```python
from build123d import *

# Parameters (mm, degrees)
Y_KSEKLIK_EKSTR_ZYON1_DEPTH = 500
RADYUS1_R                   = 2
IZIM2_R                     = 4.25
KES_EKSTR_ZYON1_DEPTH       = 10


with BuildPart() as part:
    # Çizim1 → Yükseklik-Ekstrüzyon1 (new body)
    with BuildSketch(Plane.XY):
        Polygon((0, 0), (65, 0), (65, 4), (60, 4), (60, 8), (55, 8), (55, 4), (10, 4), (10, 8), (5, 8), (5, 4), (0, 4), align=None)
    extrude(amount=-Y_KSEKLIK_EKSTR_ZYON1_DEPTH)

    # Radyus1
    radyus1_edges = [part.edges().sort_by_distance(p)[0] for p in [
        (5, 8, -250),
        (10, 8, -250),
        (55, 8, -250),
        (60, 8, -250),
    ]]
    fillet(radyus1_edges, radius=RADYUS1_R)

    # Çizim2 → Kes-Ekstrüzyon1 (cut)
    with BuildSketch(Plane.XZ):
        with Locations(Location((30, -40, 0), (0, 0, 270))):
            Circle(IZIM2_R)
        with Locations(Location((30, -180, 0), (0, 0, 270))):
            Circle(IZIM2_R)
        with Locations(Location((30, -320, 0), (0, 0, 270))):
            Circle(IZIM2_R)
        with Locations(Location((30, -460, 0), (0, 0, 270))):
            Circle(IZIM2_R)
    extrude(amount=-KES_EKSTR_ZYON1_DEPTH, mode=Mode.SUBTRACT)


solid = part.part
```
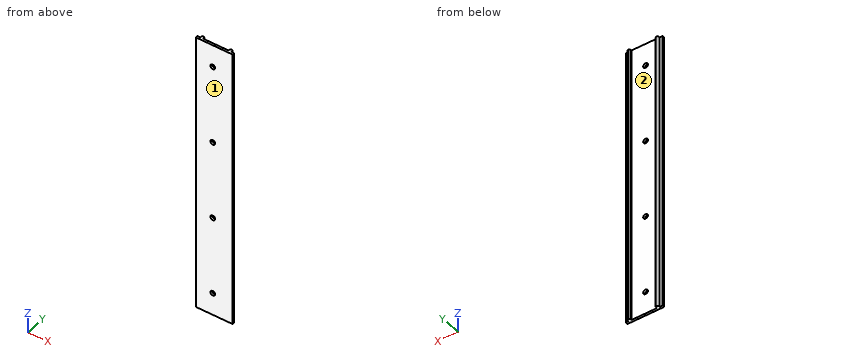
Verification items for the finished model (mm, model axes). Face numbers are marked on the shaded views. Round coordinates to 2 decimals unless told otherwise and drop trailing zeros. Order: outer loops, then holes, each group sorted by start corner. A loop starts at its lowest first (then second) coordinate and runs counter-clockwise, first axis right, second up. Notation, with made-up numbers: (54, -38) - (88, -38) arc R32 cw to (88, -12) - close; hole circle Ø4 at (32.25, -11.75). An arc over 180 degrees is marked (long way). Use CSV: the item, a comma, the result in double quotes. Start each with the question number.
1) Section check B-B, the plane z = -105.5. Record the cut outline in (x, y), plus the area to 3 significant figures.
2) Section check A-A, the plane z = -180. Record the cut outline in (x, y).
3) Section check C-C, the plane x = 14.5. Record the cut outline in (y, z), plus the area to 3 significant figures.
4) Go/stop test with flat-tipped pins: P1, Ø22.5, axis at x = 33.5, z = -310, coming from the +Y side; P2, Ø0.6, axis at y = 4.5, z = -203, coming from the -X side; P3, Ø1, axis at x = 48, y = 6, coming from the +Z side; P4, Ø5.5, axis at x = 2.5, z = -332.5, coming from the +Y side. Record where each tip stops, or that it passes through.
5) Mould release check, pull along X, two halves, no side actions. Record for the marked faces 1 and 2: +X half, -X half, draft (parallel to the pull), parting line (faces both ways), or undercut.
6) Thickness scan on L1, parallel to X at y = 6.25, z = -186; L2, parallel to X at y = 3, z = -460; L3, parallel to Y at x = 22, z = -166. Record the ranges inside material, lowest first.
Answers:
1,outline,"(0, 0) - (65, 0) - (65, 4) - (60, 4) - (60, 6) arc R2 ccw to (58, 8) - (57, 8) arc R2 ccw to (55, 6) - (55, 4) - (10, 4) - (10, 6) arc R2 ccw to (8, 8) - (7, 8) arc R2 ccw to (5, 6) - (5, 4) - (0, 4) - close"
1,area,"297 mm²"
2,outline,"(0, 0) - (25.75, 0) - (25.75, 4) - (10, 4) - (10, 6) arc R2 ccw to (8, 8) - (7, 8) arc R2 ccw to (5, 6) - (5, 4) - (0, 4) - close; (34.25, 0) - (65, 0) - (65, 4) - (60, 4) - (60, 6) arc R2 ccw to (58, 8) - (57, 8) arc R2 ccw to (55, 6) - (55, 4) - (34.25, 4) - close"
3,outline,"(0, -500) - (4, -500) - (4, 0) - (0, 0) - close"
3,area,"2,000 mm²"
4,P1,"stops at y = 4"
4,P2,"stops at x = 5"
4,P3,"passes through"
4,P4,"stops at y = 6.97"
5,face 1,"draft"
5,face 2,"undercut"
6,L1,"x = 5.02 to 9.98, 55.02 to 59.98"
6,L2,"x = 0 to 25.75, 34.25 to 65"
6,L3,"y = 0 to 4"
